from build123d import *

# Parameters (mm, degrees)
BOSS_EXTRUDE1_DEPTH = 50


with BuildPart() as part:
    # Sketch1 → Boss-Extrude1 (new body)
    with BuildSketch(Plane(origin=(0, 0, 0), x_dir=(1, 0, 0), z_dir=(0, 1, 0))):
        Polygon((0, 30), (0, 0), (0.000186337, -0.03343628), (3, 0), (3, 30), align=None)
        with BuildLine():
            Line((0.000186337, -0.03343628), (3, 0))
            add(Edge.make_bspline(
                [(3, 0), (3.139918652, -12.553127515), (-7.554025616, -14.764008615)],
                knots=[0, 0, 0, 1, 1, 1], degree=2))
            Line((-7.554025616, -14.764008615), (-29.724787296, -19.341198123))
            Line((-29.724787296, -19.341198123), (-33.586790943, -19.341198123))
            Line((-33.586790943, -19.341198123), (-8.16140534, -11.826136958))
            add(Edge.make_bspline(
                [(0.000186337, -0.03343628), (0.005239929, -0.486831056), (-0.009475768, -1.417335062), (-0.137351147, -3.087884204), (-0.471550564, -4.947811199), (-1.116797216, -6.782204669), (-1.973725508, -8.269549477), (-3.042888675, -9.477251715), (-4.37173122, -10.472028768), (-5.764833241, -11.143024266), (-7.059525511, -11.570636997), (-7.798848397, -11.751181425), (-8.16140534, -11.826136958)],
                knots=[0, 0, 0, 0, 0.0625, 0.125, 0.25, 0.375, 0.5, 0.625, 0.75, 0.875, 0.9375, 1, 1, 1, 1], degree=3))
        make_face()
    extrude(amount=BOSS_EXTRUDE1_DEPTH)


solid = part.part
Build history of the part. All positions in model axes, mm. A direction names the side the tool comes from. Give positions to 0.01 mm unless a question says otherwise; leave off trailing zeros. Order: outer loops, then holes, each group sorted by start corner. A loop starts at its lowest first (then second) coordinate and runs counter-clockwise, first axis right, second up. Notation, with made-up numbers: M -26,19 L 13,19 A18 ccw 13,46 Z; hole C 86,81 d9. An arc over 180 degrees is marked long. Put each result on its own line as item: value.
Item 1: Cut at B-B on x = -26. Write the cut outline in (y, z), then the cut area to 3 significant figures.
Results are:
outline: M 0,17.1 L 50,17.1 L 50,18.57 L 0,18.57 Z
area: 73.7 mm2
Item 2: Drop flat-ended pins along their axis: pin 1 Ø6 at (x, y) = (-17, 14.5) entering from -Z; pin 2 Ø10 at (x, y) = (-21, 19.5) entering from -Z; pin 3 Ø2 at (x, y) = (-13, 14) entering from -Z. Give the stop position or say it passes through.
Results are:
pin 1: z = 13.55
pin 2: z = 14.14
pin 3: z = 12.96
Item 3: Cut at A-A on z = -3. Write the cut outline in (x, y), then the cut area to 3 significant figures.
Results are:
outline: M 0,0 L 3,0 L 3,50 L 0,50 Z
area: 150 mm2
Item 4: Which spindle directions (+Z, -Z, +X, -X, +Y, -Y) get a long thin tool onto all of the face, cutting with end or side? Do faces 1 (the face through (-18.48, 24.65, 17.02)), 2 (the face through (0, 25, -15)). Say none if no direction does.
Results are:
face 1: +Z, +X, +Y, -Y
face 2: -Z, -X, +Y, -Y
Item 5: Wall check: probe 1 along X at (y, z) = (46.5, -15); probe 2 along Z at (x, y) = (-18, 22); probe 3 along X at (y, z) = (28, 9). Give the ranges that are in metal, low to high.
Results are:
probe 1: 0 to 3
probe 2: 14.73 to 16.92
probe 3: -2.64 to 1.05
